```python
from build123d import *

# Parameters (mm, degrees)
SKETCH2_W           = 50
SKETCH2_H           = 50
BOSS_EXTRUDE1_DEPTH = 10
SKETCH4_R           = 2.1
CUT_EXTRUDE1_DEPTH  = 4.57
SKETCH5_W           = 20
SKETCH5_H           = 20
CUT_EXTRUDE2_DEPTH  = 5.43


with BuildPart() as part:
    # Sketch2 → Boss-Extrude1 (new body)
    with BuildSketch(Plane(origin=(0, 0, 0), x_dir=(1, 0, 0), z_dir=(0, 1, 0))):
        Rectangle(SKETCH2_W, SKETCH2_H)
    extrude(amount=BOSS_EXTRUDE1_DEPTH)

    # Sketch4 → Cut-Extrude1 (cut)
    with BuildSketch(Plane(origin=(0, 10, 0), x_dir=(1, 0, 0), z_dir=(0, 1, 0))):
        Circle(SKETCH4_R)
        with Locations((6.35, 6.35)):
            Circle(SKETCH4_R)
        with Locations((-6.35, 6.35)):
            Circle(SKETCH4_R)
        with Locations((-6.35, -6.35)):
            Circle(SKETCH4_R)
        with Locations((6.35, -6.35)):
            Circle(SKETCH4_R)
    extrude(amount=-CUT_EXTRUDE1_DEPTH, mode=Mode.SUBTRACT)

    # Sketch5 → Cut-Extrude2 (cut)
    with BuildSketch(Plane.XZ):
        Rectangle(SKETCH5_W, SKETCH5_H)
    extrude(amount=-CUT_EXTRUDE2_DEPTH, mode=Mode.SUBTRACT)


solid = part.part
```
Source: CAD feature listing. Evaluate the final solid. Frame: model axes, mm. A direction names the side the tool comes from. Round coordinates to 2 decimals unless told otherwise and drop trailing zeros. Loops run counter-clockwise (first coordinate to the right, second up) from the corner with the lowest first, then second, coordinate; pieces in that order, holes last. Notation, with made-up numbers: M 74.25,-27 L 88.25,-27 A18 ccw 88.25,-2 Z; hole C 39.5,11 d4. An arc over 180 degrees is marked long. Use a Markdown table: item, result. Add a question column.
1. Set-up query: faces 1 (the flat face through (0, 3, 10)), 2 (the flat face through (0, 0, -11)). Return all of +Z, -Z, +X, -X, +Y, -Y with unobstructed straight access to the full face (end or side cutting, diameter ignored); none if empty.
2. Cut plane D-D, the plane y = 1. Output: boundary loops of the cut face in (x, z).
3. Cut plane A-A, the plane z = 6.35. Output: boundary loops of the cut face in (x, y).
4. Cut plane B-B, the plane x = -6.35. Output: boundary loops of the cut face in (y, z), and give its area (3 significant figures).
5. Pull-direction query (Z, two-part tool) for faces 3 (the flat face through (-25, 5, 0)), 4 (the flat face through (0, 5, 25)), 5 (the flat face through (-0.1, 5.43, 2.4)); classes: +Z half, -Z half, draft (parallel to the pull), parting line (faces both ways), or undercut.
6. Cut plane C-C, the plane x = 0. Output: boundary loops of the cut face in (y, z), and give its area (3 significant figures).
7. Contact query for a flat-ended pin moving along its axis: pin 1 (5.5 mm diameter, centred on x = -6.35, z = 6.35, fed in from -Y). Output: stop coordinate, or through.
8. Ray query, line 1 along Z through (x, y) = (6.35, 7.35); line 2 along X through (y, z) = (2.5, 1.5). Return the intervals inside material, ascending. Write a range as [from, to].
Solution:
| question | item | result |
|---|---|---|
| 1 | face 1 | -Y |
| 1 | face 2 | +Z, -Z, +X, -X, -Y |
| 2 | outline | M -25,-25 L 25,-25 L 25,25 L -25,25 Z; hole M -10,-10 L 10,-10 L 10,10 L -10,10 Z |
| 3 | outline | M -25,0 L -10,0 L -10,5.43 L -8.45,5.43 L -8.45,10 L -25,10 Z; M -4.25,5.43 L 4.25,5.43 L 4.25,10 L -4.25,10 Z; M 8.45,5.43 L 10,5.43 L 10,0 L 25,0 L 25,10 L 8.45,10 Z |
| 4 | outline | M 0,-25 L 10,-25 L 10,-8.45 L 5.43,-8.45 L 5.43,-10 L 0,-10 Z; M 0,10 L 5.43,10 L 5.43,8.45 L 10,8.45 L 10,25 L 0,25 Z; M 5.43,-4.25 L 10,-4.25 L 10,4.25 L 5.43,4.25 Z |
| 4 | area | 353 mm2 |
| 5 | face 3 | draft |
| 5 | face 4 | +Z half |
| 5 | face 5 | undercut |
| 6 | outline | M 0,-25 L 10,-25 L 10,-2.1 L 5.43,-2.1 L 5.43,-10 L 0,-10 Z; M 0,10 L 5.43,10 L 5.43,2.1 L 10,2.1 L 10,25 L 0,25 Z |
| 6 | area | 372 mm2 |
| 7 | pin 1 | stops at y = 5.43 |
| 8 | line 1 | z = [-25, -8.45], [-4.25, 4.25], [8.45, 25] |
| 8 | line 2 | x = [-25, -10], [10, 25] |
